Autodesk Inventor part; units mm, degrees
ref_plane "Work Plane3" through (0, 17.1421, -87.8579) normal (0, 1, 0) x (-1, 0, 0)
ref_plane "YZ Plane" through (0, 0, 0) normal (1, 0, 0) x (0, 1, 0)
ref_plane "XY Plane" through (0, 0, 0) normal (0, 0, 1) x (1, 0, 0)
sketch "Sketch1" plane through (0, 0, 0) normal (1, 0, 0) x (0, 1, 0)
  line L0 (0, 105) -> (55, 50)
  line L1 (55, 50) -> (55, -50)
  line L2 (55, -50) -> (0, -105)
  line L3 (0, 105) -> (0, -115) construction
  line L4 (0, -76.7157) -> (35, -41.7157)
  line L5 (35, -41.7157) -> (35, 41.7157)
  line L6 (35, 41.7157) -> (0, 76.7157)
  line L7 (0, -115) -> (0, -76.7157)
  line L8 (0, 76.7157) -> (0, 105)
  point P0 (0, 0)
  point P1 (55, 0)
  point P2 (0, -5)
  point P3 (35, 0)
  point P4 (0, -105)
  dimension "d0" = 210
  dimension "d2" = 45
  dimension "d3" = 20
  dimension "d4" = 35
  dimension "d5" = 20
extrude "Extrusion1" add sketch "Sketch1" along normal mid plane 25
chamfer "Chamfer1" distance 5 angle 45 6 edges at (-12.5, 27.5, -77.5) (-12.5, 55, 0) (-12.5, 27.5, 77.5) (12.5, 27.5, 77.5) (12.5, 55, 0) (12.5, 27.5, -77.5)
chamfer "Chamfer2" distance 5 angle 45 6 edges at (7.5, 27.5, 77.5) (-7.5, 27.5, 77.5) (-7.5, 55, 0) (7.5, 55, 0) (7.5, 27.5, -77.5) (-7.5, 27.5, -77.5)
fillet "Fillet1" radius 3 6 edges at (12.5, 25, 72.9289) (12.5, 50, 0) (12.5, 25, -72.9289) (-12.5, 25, -72.9289) (-12.5, 50, 0) (-12.5, 25, 72.9289)
fillet "Fillet2" radius 3 6 edges at (-12.5, 17.5, -59.2157) (-12.5, 35, 0) (-12.5, 17.5, 59.2157) (12.5, 17.5, 59.2157) (12.5, 35, 0) (12.5, 17.5, -59.2157)
sketch "Sketch2" plane through (-2.5, 0, 105) normal (0, -1, 0) x (1, 0, 0)
  line L0 (-7, -181.7157) -> (12, -181.7157)
  line L1 (0, -210) -> (5, -210)
  point P0 (2.5, -105)
  point P1 (2.5, -195.8579)
  point P2 (2.5, -181.7157)
  point P3 (2.5, -181.7157)
  point P4 (2.5, -210)
  dimension "d20" = 14.1421
  dimension "d22" = 28.2843
hole "Hole1" at (0, 0, -90.8579) direction (0, 1, 0) diameter 6 end through all
ref_plane "Work Plane3" through (0, 17.1421, -87.8579) normal (0, 1, 0) x (-1, 0, 0)
sketch "Sketch6" plane through (0, 17.1421, -87.8579) normal (0, 1, 0) x (-1, 0, 0)
  arc A0 (-2.5, -4.6583) -> (2.5, -4.6583) centre (0, -3) ccw
  circle A1 centre (0, -3) radius 6
  point P0 (0, 87.8579)
  dimension "d37" = 12
extrude "Extrusion4" cut sketch "Sketch6" along normal blind 3 and the other way blind 6.5
mirror "Mirror2" about plane through (0, 0, 0) normal (0, 0, 1) of "Extrusion4", "Hole1"
properties part number "Handle"
Read the model definition and answer for the solid it produces. Units are mm, in the model's axes. A direction names the side the tool comes from. Coordinates: 2 decimals unless noted, no trailing zeros. Loops run counter-clockwise (first coordinate to the right, second up) from the corner with the lowest first, then second, coordinate; pieces in that order, holes last. Notation, with made-up numbers: (27, 48.25) -> (49, 48.25) arc R9 ccw to (49, 65.25) -> close; hole circle Ø2 at (39, 31). An arc over 180 degrees is marked (long way). Answer in a Markdown table with one row per item.
Item 1: A cutting plane is placed at C-C on y = 7.5. Give the number of separate pieces and of enclosed holes in the cut face, plus the area to 3 significant figures.
Returned:
| item | result |
|---|---|
| separate pieces | 2 |
| enclosed holes | 2 |
| area | 1,220 mm^2 |
Item 2: A cutting plane is placed at B-B on z = -2.5. Determine the outline of the cut face in (x, y), plus the area to 3 significant figures.
Returned:
| item | result |
|---|---|
| outline | (-12.5, 38) arc R3 ccw to (-9.5, 35) -> (9.5, 35) arc R3 ccw to (12.5, 38) -> (12.5, 48.76) arc R3 ccw to (11.62, 50.88) -> (11.04, 51.46) -> (2.5, 55) -> (-2.5, 55) -> (-11.04, 51.46) -> (-11.62, 50.88) arc R3 ccw to (-12.5, 48.76) -> close |
| area | 453 mm^2 |
Item 3: For a pull along Z with two mould halves and no side action, classify faces 4 (the cylindrical face through (-12.278, 25.096, 72.677)), 5 (the flat face through (-0.133, 17.745, 58.971)), 6 (the flat face through (0, 55, 1)) as released by +Z, released by -Z, zero draft, split by the parting line, or undercut.
Returned:
| item | result |
|---|---|
| face 4 | released by +Z |
| face 5 | undercut |
| face 6 | zero draft |
Item 4: For faces 1 (the flat face through (11.33, 25.88, 73.7)), 2 (the flat face through (0, 35, -1)), 3 (the cylindrical face through (11.6, 17.75, -60.18)), determine the directions among +Z, -Z, +X, -X, +Y, -Y from which every point of the face is accessible in a straight line to the end or side of a thin tool.
Returned:
| item | result |
|---|---|
| face 1 | +Z, +X, +Y |
| face 2 | +X, -X, -Y |
| face 3 | +X, -Y |
Item 5: Straight lines are drawn through the part: line 1 along Z through (x, y) = (0, 3.25); line 2 along Z through (x, y) = (0, 4.75); line 3 along Z through (x, y) = (0, 18). For each, find the intervals that lie inside material, in ascending order. Write a range as [from, to].
Returned:
| item | result |
|---|---|
| line 1 | z = [-101.75, -93.86], [-87.86, -73.47], [73.47, 87.86], [93.86, 101.75] |
| line 2 | z = [-100.25, -93.86], [-87.86, -71.97], [71.97, 87.86], [93.86, 100.25] |
| line 3 | z = [-84.86, -58.72], [58.72, 84.86] |
Item 6: Each of these flat-tipped pins is pushed along its axis until it touches: P1, Ø6, axis at y = 35, z = -24.5, coming from the +X side; P2, Ø10.5, axis at x = -0.5, z = -88, coming from the +Y side; P3, Ø5, axis at x = 4, z = -58.5, coming from the -Y side; P4, Ø8, axis at x = 0, z = -90.86, coming from the +Y side. Where does it stop, or does it pass through?
Returned:
| item | result |
|---|---|
| P1 | stops at x = 12.5 |
| P2 | stops at y = 22.25 |
| P3 | stops at y = 15.72 |
| P4 | stops at y = 10.64 |
Item 7: A cutting plane is placed at A-A on x = 0. Determine the outline of the cut face in (y, z).
Returned:
| item | result |
|---|---|
| outline | (0, -105) -> (10.64, -94.36) -> (10.64, -93.86) -> (0, -93.86) -> close; (0, -87.86) -> (10.64, -87.86) -> (10.64, -84.86) -> (20.14, -84.86) -> (55, -50) -> (55, 50) -> (20.14, 84.86) -> (10.64, 84.86) -> (10.64, 87.86) -> (0, 87.86) -> (0, 76.72) -> (35, 41.72) -> (35, -41.72) -> (0, -76.72) -> close; (0, 93.86) -> (10.64, 93.86) -> (10.64, 94.36) -> (0, 105) -> close |
